Source: CAD feature listing. Evaluate the final solid. Frame: model axes, mm. Give positions to 0.01 mm unless a question says otherwise; leave off trailing zeros. Order: outer loops, then holes, each group sorted by start corner. A loop starts at its lowest first (then second) coordinate and runs counter-clockwise, first axis right, second up. Notation, with made-up numbers: M -15,-40 L 34,-40 A32 ccw 34,-10 Z; hole C 80,34 d4. An arc over 180 degrees is marked long. Answer as a JSON object with one key per item and string values. Group by question number.
1. Section query B-B (x = -9). Output: boundary loops of the cut face in (y, z), plus the area to 3 significant figures.
2. Material intervals for L1, parallel to Y at x = 6.5, z = -76, sorted ascending. Write a range as [from, to].
3. Section query A-A (z = -64). Output: boundary loops of the cut face in (x, y).
4. Pin query (flat end, axial travel): P1, Ø19, axis at x = 9.5, y = -554.5, coming from the -Z side. Return the tip coordinate at first contact, or that it passes through.
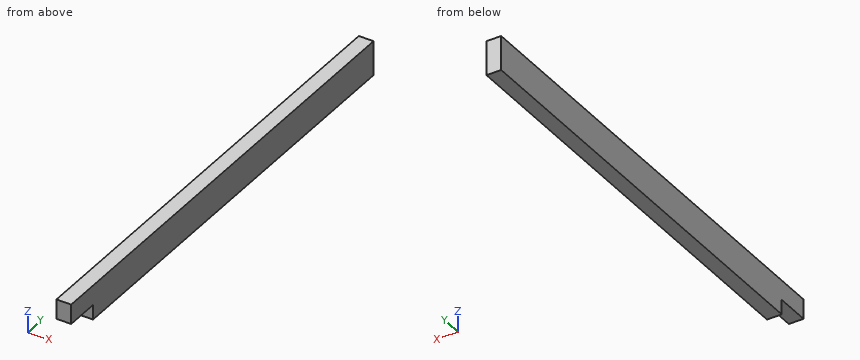
from build123d import *

# Parameters (mm, degrees)
F0_W     = 38.1
F0_H     = 1143
F1_DEPTH = 88.9
F0_H_2   = 88.9
F2_DEPTH = 50.8


with BuildPart() as f1:
    # F0 (on Top) → F1 (new body)
    with BuildSketch(Plane.XY):
        with Locations((0, 44.45)):
            Rectangle(F0_W, F0_H)
    extrude(amount=-F1_DEPTH)

    # F0 (on Top) → F2 (join)
    with BuildSketch(Plane.XY):
        with Locations((0, -571.5)):
            Rectangle(F0_W, F0_H_2)
    extrude(amount=-F2_DEPTH)


solid = f1.part
Answer sheet:
{
 "1": {"outline": "M -615.95,-50.8 L -527.05,-50.8 L -527.05,-88.9 L 615.95,-88.9 L 615.95,0 L -615.95,0 Z", "area": "106,000 mm^2"},
 "2": {"L1": "[-527.05, 615.95]"},
 "3": {"outline": "M -19.05,-527.05 L 19.05,-527.05 L 19.05,615.95 L -19.05,615.95 Z"},
 "4": {"P1": "z = -50.8"}
}
